Part print with two shaded views. Sizes in mm from the minimum x, y, z corner. A direction names the side the tool comes from. Give positions to 0.01 mm unless a question says otherwise; leave off trailing zeros. Write each loop counter-clockwise with the first axis right and the second up, starting at its lowest first coordinate (ties: lowest second). Pieces come first, ordered by that corner, then holes. Notation, with made-up numbers: (-10, -14.5) - (15, -14.5) arc R24 cw to (15, -4.5) - close; hole circle Ø11 at (8, 17). An arc over 180 degrees is marked (long way). One line per item, written item: value. Start each with the question number.
(1) Cut at A-A, the plane x = 13.5. List the corners of the cut face in (y, z) (1 decimal).
(2) Probe L1, parallel to X at y = 10, z = 12; L2, parallel to Y at x = 13.5, z = 13.25; L3, parallel to Z at x = 18.5, y = 16 (1 decimal). List the from-to ranges inside material, lowest first.
(3) Cut at C-C, the plane z = 2.25. List the corners of the cut face in (x, y), and give its area (3 significant figures).
(4) 3-axis set-ups, long thin cutter, end or side, ignore diameter. For the marked faces 1, 2 and 3: which of +Z, -Z, +X, -X, +Y, -Y reach the whole face in a straight line?
(5) Drop flat-ended pins along their axis: P1, Ø1.5, axis at y = 45.5, z = 9.5, coming from the +X side (1 decimal); P2, Ø4.5, axis at y = 18.5, z = 8, coming from the +X side; P3, Ø7, axis at x = 13, y = 24, coming from the +Z side. Give the stop position or say it passes through.
(6) Cut at B-B, the plane y = 16. List the corners of the cut face in (x, z) (1 decimal), and give its area (3 significant figures).
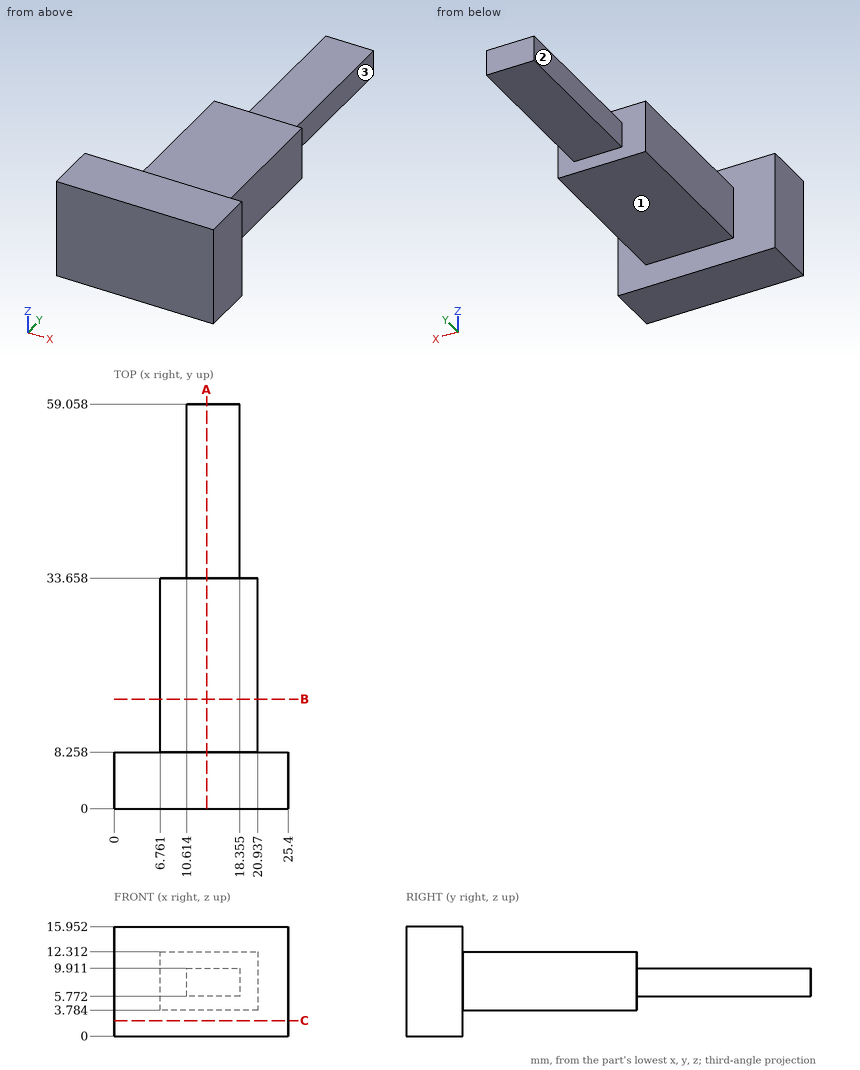
Answers follow:
1. outline: (0, 0) - (8.3, 0) - (8.3, 3.8) - (33.7, 3.8) - (33.7, 5.8) - (59.1, 5.8) - (59.1, 9.9) - (33.7, 9.9) - (33.7, 12.3) - (8.3, 12.3) - (8.3, 16) - (0, 16) - close
2. L1: x = 6.76 to 20.94
2. L2: y = 0 to 8.26
2. L3: z = 3.8 to 12.3
3. outline: (0, 0) - (25.4, 0) - (25.4, 8.26) - (0, 8.26) - close
3. area: 210 mm²
4. face 1: -Z, +X, -X, +Y
4. face 2: +Z, -Z, -X, +Y
4. face 3: +Z, -Z, +X, +Y
5. P1: stops at x = 18.4
5. P2: stops at x = 20.94
5. P3: stops at z = 12.31
6. outline: (6.8, 3.8) - (20.9, 3.8) - (20.9, 12.3) - (6.8, 12.3) - close
6. area: 121 mm²
